Can you work these out from the model? Positions are in its coordinate system, mm. A direction names the side the tool comes from. Coordinates: 2 decimals unless noted, no trailing zeros. Write each loop counter-clockwise with the first axis right and the second up, starting at its lowest first coordinate (ties: lowest second). Pieces come first, ordered by that corner, then holes. Notation, with made-up numbers: (6.5, 6) -> (37.5, 6) arc R28 ccw to (37.5, 44) -> close; hole circle Ø4 at (-17, 65). An arc over 180 degrees is marked (long way). Answer as CSV lines item,"result". Start each with the question number.
Autodesk Inventor part; units mm, degrees
ref_plane "YZ Plane" through (0, 0, 0) normal (1, 0, 0) x (0, 1, 0)
ref_plane "XZ Plane" through (0, 0, 0) normal (0, 1, 0) x (-1, 0, 0)
ref_plane "XY Plane" through (0, 0, 0) normal (0, 0, 1) x (1, 0, 0)
sketch "Boceto1" plane through (0, 0, 0) normal (0, 0, 1) x (1, 0, 0)
  line L0 (0, 0) -> (105, 0)
  line L1 (105, 0) -> (105, 55)
  line L2 (105, 55) -> (0, 0)
  line L3 (105, 55) -> (90, 55)
  line L4 (90, 55) -> (0, 0)
  line L5 (0, 0) -> (70, 0)
  line L6 (70, 0) -> (90, 55)
  dimension "d0" = 105
  dimension "d1" = 55
  dimension "d4" = 15
  dimension "d10" = 70
extrude "Extrusión1" add sketch "Boceto1" along normal blind 10 contours L6 L2 L1 L0 | L6 L3 L2
sketch "Boceto2" plane through (0, 0, 10) normal (0, 0, 1) x (1, 0, 0)
  line L0 (-10.0369, 16.82) -> (-5.1631, 16.82)
  line L1 (-1.5564, 16.82) -> (-5.1631, 16.82)
  line L2 (-1.5564, 16.82) -> (105, 16.82)
  line L3 (105, 0) -> (105, 55)
  line L4 (105, 55) -> (90, 55)
  line L5 (70, 0) -> (105, 0)
  line L6 (100, 5) -> (14.5727, 5)
  line L7 (90, 55) -> (70, 0)
  line L8 (105, 55) -> (105, 42.8)
  line L9 (105, 55) -> (117.2, 55) construction
  line L10 (70, 0) -> (105, 0)
  line L11 (105, 0) -> (105, 16.82)
  line L12 (105, 0) -> (105, 55)
  line L13 (105, 16.82) -> (100, 16.82)
  line L14 (100, 16.82) -> (94.1, 16.82)
  line L15 (94.1, 16.82) -> (94.1, 25.02)
  line L16 (94.1, 25.02) -> (100, 25.02)
  line L17 (100, 25.02) -> (100, 16.82)
  line L18 (105, 42.8) -> (100, 42.8)
  line L19 (100, 42.8) -> (91.8, 42.8)
  line L20 (91.8, 42.8) -> (91.8, 51)
  line L21 (91.8, 51) -> (100, 51)
  line L22 (100, 51) -> (100, 42.8)
  line L23 (100, 16.82) -> (91.8, 16.82)
  line L24 (91.8, 16.82) -> (91.8, 25.02)
  line L25 (91.8, 25.02) -> (100, 25.02)
  line L26 (100, 25.02) -> (100, 16.82)
  point P0 (0, 0)
  point P1 (94.1, 16.82)
  point P2 (100, 25.02)
  point P3 (91.8, 16.82)
  point P4 (105, 25.02)
  point P5 (162.8, 25.02)
  point P6 (162.8, 16.82)
  dimension "d22" = 90
  dimension "d25" = 8.2
  dimension "d26" = 12.2
  dimension "d27" = 8.2
  dimension "d28" = 8.2
  dimension "d31" = 8.2
extrude "Extrusión2" cut sketch "Boceto2" against normal through all contours L24 L25 L15 L2 | L15 L16 L17 L2 | L19 L20 L21 L22
sketch "Boceto3" plane through (70, 0, 0) normal (0, -1, 0) x (1, 0, 0)
  line L0 (21.8, 10) -> (21.8, 0)
  line L1 (0, 10) -> (35, 10)
  line L2 (0, 0) -> (35, 0)
  line L3 (35, 0) -> (35, 10)
  line L4 (0, 10) -> (0, 0)
  point P0 (-70, 0)
extrude "Extrusión3" add sketch "Boceto3" along normal blind 10
sketch "Boceto4" plane through (0, 0, 10) normal (0, 0, 1) x (1, 0, 0)
  circle A0 centre (100, -5) radius 2.1
  circle A1 centre (75, -5) radius 2.1
  point P0 (0, 0)
hole "Agujero1" at (75, -5, 10) at (100, -5, 10) direction (0, 0, -1) diameter 3.2 depth 10
shell "Vaciado1" thickness 6 removed faces 2 at (88.9333, 2.8793, 10) at (88.9333, 2.8793, 0)
fillet "Empalme1" radius 6 2 edges at (99, 10.82, 5) (85.8, 10.82, 5)
properties part number "Soporte lateral"
Q1. Imagine slicing it at D-D (y = 14.5). Write out the boundary of the cut face in (x, z).
Q2. I need wall thicknesses on L1, parallel to X at y = -5, z = 1.5; L2, parallel to X at y = 22, z = 6.75; L3, parallel to Y at x = 95, z = 6.5. Which ranges of each line are inside material? Lowest first, please.
Q3. Which directions (+Z, -Z, +X, -X, +Y, -Y) give clear straight access to the entire face, cutting with the end or side of a thin tool? Please do faces 1 (the face through (98, 55, 5)), 2 (the face through (94.577, 0.325, 4.93)).
Q4. Imagine slicing it at A-A (y = -5). Write out the boundary of the cut face in (x, z).
Q5. Imagine slicing it at B-B (z = 3.25). Write out the boundary of the cut face in (x, y).
Q6. If we mould it in two halves opening along X, with no side actions, what happens to faces 3 (the face through (91, 23, 0)), 4 (the face through (105, 22, 5)), 5 (the face through (91.8, 47, 5))? For each: released by +X, released by -X, zero draft, split by the parting line, or undercut.
Q7. For pin 1 (4.5 mm diameter, centred on y = 34, z = 3, fed in from -X); pin 2 (2.5 mm diameter, centred on x = 75, y = -5, fed in from +Z); pin 3 (1.8 mm diameter, centred on y = 4, z = 3, fed in from -X), each with a flat end and sliding along its axis, tell me the tip position at first contact or that it passes through.
Q8. Imagine slicing it at C-C (x = 75). Write out the boundary of the cut face in (y, z), then the cut area to 4 significant figures.
Entries:
1,outline,"(75.27, 0) -> (81.66, 0) -> (81.66, 10) -> (75.27, 10) -> close; (86.27, 0) -> (105, 0) -> (105, 10) -> (86.27, 10) -> close"
2,L1,"70 to 73.4, 76.6 to 98.4, 101.6 to 105"
2,L2,"78 to 84.38, 85.8 to 91.8, 100 to 105"
2,L3,"-10 to 0.72, 10.48 to 16.82, 25.02 to 31.02, 36.8 to 42.8, 51 to 55"
3,face 1,"+Z, -Z, +X, -X, +Y"
3,face 2,"+Z, -Z"
4,outline,"(70, 0) -> (73.4, 0) -> (73.4, 10) -> (70, 10) -> close; (76.6, 0) -> (98.4, 0) -> (98.4, 10) -> (76.6, 10) -> close; (101.6, 0) -> (105, 0) -> (105, 10) -> (101.6, 10) -> close"
5,outline,"(70, -10) -> (105, -10) -> (105, 55) -> (90, 55) -> (70, 0) -> close; hole circle Ø3.2 at (75, -5); hole (77.21, 2.27) arc R7.6 cw to (82.53, -4) -> (92.47, -4) arc R7.6 cw to (99, 2.53) -> (99, 4.82) arc R6 ccw to (93, 10.82) -> (91.8, 10.82) arc R6 cw to (85.8, 16.82) -> (85.8, 25.89) -> close; hole (87.66, 31.02) -> (99, 31.02) -> (99, 36.8) -> (89.77, 36.8) -> close; hole (91.8, 16.82) -> (100, 16.82) -> (100, 25.02) -> (91.8, 25.02) -> close; hole (91.8, 42.8) -> (100, 42.8) -> (100, 51) -> (91.8, 51) -> close; hole circle Ø3.2 at (100, -5)"
6,face 3,"zero draft"
6,face 4,"released by +X"
6,face 5,"undercut"
7,pin 1,"x = 81.55"
7,pin 2,"through"
7,pin 3,"x = 71.13"
8,outline,"(-10, 0) -> (-6.6, 0) -> (-6.6, 10) -> (-10, 10) -> close; (-3.4, 0) -> (13.75, 0) -> (13.75, 10) -> (-3.4, 10) -> close"
8,area,"205.5 mm2"
